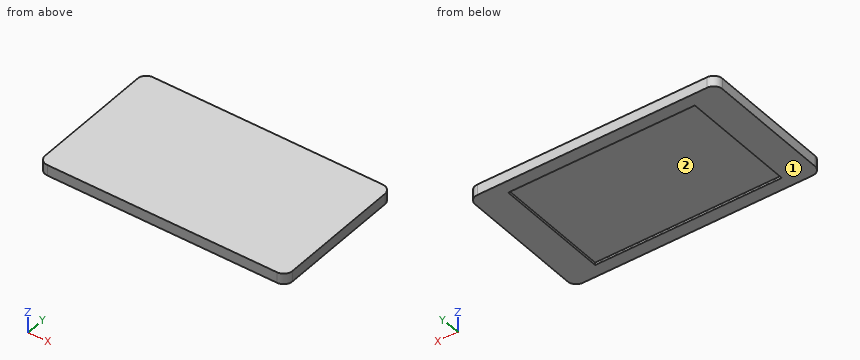
```python
from build123d import *

# Parameters (mm, degrees)
SKETCH1_W           = 200
SKETCH1_H           = 114
BOSS_EXTRUDE1_DEPTH = 8.7
SKETCH1_3_W         = 151
SKETCH1_3_H         = 94
CUT_EXTRUDE1_DEPTH  = 2
FILLET1_R           = 7


with BuildPart() as part:
    # Sketch1 → Boss-Extrude1 (new body)
    with BuildSketch(Plane.XY):
        with Locations((0, 57)):
            Rectangle(SKETCH1_W, SKETCH1_H)
    extrude(amount=BOSS_EXTRUDE1_DEPTH)

    # Sketch1<3> → Cut-Extrude1 (cut)
    with BuildSketch(Plane.XY):
        with Locations((0, 57)):
            Rectangle(SKETCH1_3_W, SKETCH1_3_H)
    extrude(amount=CUT_EXTRUDE1_DEPTH, mode=Mode.SUBTRACT)

    # Fillet1
    fillet1_edges = [part.edges().sort_by_distance(p)[0] for p in [
        (-100, 0, 4.35),
        (100, 0, 4.35),
        (100, 114, 4.35),
        (-100, 114, 4.35),
    ]]
    fillet(fillet1_edges, radius=FILLET1_R)


solid = part.part
```
Design review of the part built by this model. Coordinates are the model's own, in mm. Face numbers are marked on the shaded views. Coordinates: 2 decimals unless noted, no trailing zeros. Order: outer loops, then holes, each group sorted by start corner. A loop starts at its lowest first (then second) coordinate and runs counter-clockwise, first axis right, second up. Notation, with made-up numbers: M 25,-1.5 L 33,-1.5 A26 ccw 33,37.5 Z; hole C 29.5,44.5 d3. An arc over 180 degrees is marked long. Answer as a JSON object with one key per item and string values. Group by question number.
1) Add section A-A, the plane y = 50. Write out the cut boundary in (x, z), then the cut area to 3 significant figures.
2) Add section B-B, the plane x = 15. Write out the cut boundary in (y, z), then the cut area to 3 significant figures.
3) Wall thickness on L1, parallel to Y at x = 19, z = 0.5; L2, parallel to X at y = 107.5, z = 6.5; L3, parallel to Z at x = -7.5, y = 48: over which ranges is each line inside the solid? List them lowest first.
4) Mouldability with a two-part tool opening along Y and no side actions: class the marked faces 1 and 2 as pulls with the +Y half, pulls with the -Y half, needs draft (parallel to the pull), parting line crosses it, or undercut.
Computed values:
{
 "1": {"outline": "M -100,0 L -75.5,0 L -75.5,2 L 75.5,2 L 75.5,0 L 100,0 L 100,8.7 L -100,8.7 Z", "area": "1,440 mm^2"},
 "2": {"outline": "M 0,0 L 10,0 L 10,2 L 104,2 L 104,0 L 114,0 L 114,8.7 L 0,8.7 Z", "area": "804 mm^2"},
 "3": {"L1": "y = 0 to 10, 104 to 114", "L2": "x = -99.98 to 99.98", "L3": "z = 2 to 8.7"},
 "4": {"face 1": "needs draft", "face 2": "undercut"}
}
